from build123d import *

# Parameters (mm, degrees)
FILLET1_R = 5
FILLET2_R = 2


with BuildPart() as part:
    # Sketch1 → Revolve1 (revolve)
    with BuildSketch(Plane.XY, mode=Mode.PRIVATE) as revolve1_sk:
        Polygon((6.178218081, 62.486265198), (6.178218081, 27.486265198), (16.178218081, 27.486265198), (16.178218081, 22.486265198), (8.178218081, 22.486265198), (8.178218081, -29.513734802), (6.178218081, -29.513734802), (6.178218081, -64.513734802), (2.178218081, -64.513734802), (2.178218081, 62.486265198), align=None)
    revolve(revolve1_sk.sketch.rotate(Axis((2.178218081, 62.486265198, 0), (0, -1, 0)), 180), axis=Axis((2.178218081, 62.486265198, 0), (0, -1, 0)))

    # Fillet1
    fillet1_edges = [part.edges().sort_by_distance(p)[0] for p in [
        (6.178218081, 27.486265198, 0),
    ]]
    fillet(fillet1_edges, radius=FILLET1_R)

    # Fillet2
    fillet2_edges = [part.edges().sort_by_distance(p)[0] for p in [
        (8.178218081, 22.486265198, 0),
    ]]
    fillet(fillet2_edges, radius=FILLET2_R)

    # Fillet3: read off the stored shape, not the designer's step
    # Fillet3 outline → Fillet3 (revolve)
    with BuildSketch(Plane(origin=(2.178218081, 0, 0), x_dir=(1, 0, 0), z_dir=(0, 0, 1))):
        with BuildLine():
            Line((4, -29.513734802), (4, -30.927948365))
            ThreePointArc((4, -30.927948365), (4.414213562, -29.927948365), (5.414213562, -29.513734802))
            Line((5.414213562, -29.513734802), (4, -29.513734802))
        make_face()
    revolve(axis=Axis((2.178218081, 0, 0), (0, 1, 0)))


solid = part.part
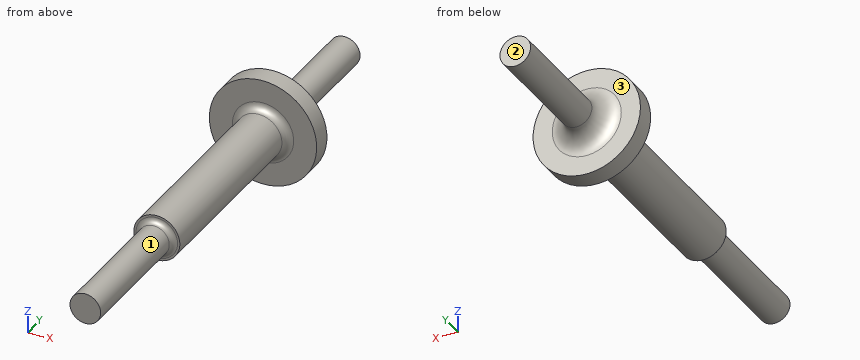
Verification items for the finished model (mm, model axes). Face numbers are marked on the shaded views. A direction names the side the tool comes from. Give positions to 0.01 mm unless a question says otherwise; leave off trailing zeros. Write each loop counter-clockwise with the first axis right and the second up, starting at its lowest first coordinate (ties: lowest second). Pieces come first, ordered by that corner, then holes. Notation, with made-up numbers: (7, 46) - (11, 46) arc R20 ccw to (11, 84) - close; hole circle Ø2 at (31, 44.5). An arc over 180 degrees is marked (long way). Answer as CSV lines item,"result". Start each with the question number.
1. Sectioned sample at C-C (z = 12). Record the boundary of the cut face in (x, y), then the cut area to 3 significant figures.
2. Sectioned sample at B-B (y = -8.5). Record the boundary of the cut face in (x, z).
3. Depth check by flat-ended pin: pin 1 (12 mm diameter, centred on y = 18, z = -1.5, fed in from -X); pin 2 (10 mm diameter, centred on y = 15, z = -5, fed in from +X); pin 3 (4 mm diameter, centred on y = 43, z = -2.5, fed in from +X); pin 4 (8 mm diameter, centred on x = 9, y = 35, fed in from +Z). Enter the tip coordinate at first touch or a pass-through.
4. Thickness scan on line 1 (Y direction, x = 12, z = -2.25); line 2 (X direction, y = 5.5, z = -0.5); line 3 (Z direction, x = 2.25, y = -11.5). Record the ranges inside material, lowest first.
5. Sectioned sample at A-A (z = 0). Record the boundary of the cut face in (x, y).
6. Set-up check for the marked faces 1, 2 and 3: record each of +Z, -Z, +X, -X, +Y, -Y from which the full face is reachable in a straight line by a thin tool's end or side.
Derived:
1,outline,"(-5.03, 22.49) - (9.39, 22.49) - (9.39, 27.49) - (-5.03, 27.49) - close"
1,area,"72.1 mm²"
2,outline,"circle Ø12 at (2.18, 0)"
3,pin 1,"x = -11.82"
3,pin 2,"x = 8.18"
3,pin 3,"x = 6.15"
3,pin 4,"z = 2.84"
4,line 1,"22.49 to 27.49"
4,line 2,"-3.8 to 8.16"
4,line 3,"-6 to 6"
5,outline,"(-11.82, 22.49) - (-5.82, 22.49) arc R2 cw to (-3.82, 20.49) - (-3.82, -29.51) - (-3.24, -29.51) arc R1.41 cw to (-1.82, -30.93) - (-1.82, -64.51) - (6.18, -64.51) - (6.18, -30.93) arc R1.41 cw to (7.59, -29.51) - (8.18, -29.51) - (8.18, 20.49) arc R2 cw to (10.18, 22.49) - (16.18, 22.49) - (16.18, 27.49) - (11.18, 27.49) arc R5 cw to (6.18, 32.49) - (6.18, 62.49) - (-1.82, 62.49) - (-1.82, 32.49) arc R5 cw to (-6.82, 27.49) - (-11.82, 27.49) - close"
6,face 1,"-Y"
6,face 2,"+Z, -Z, +X, -X, +Y"
6,face 3,"+Y"
